Geometry: final body of the model. Coordinates: model frame, mm. A direction names the side the tool comes from. Round coordinates to 2 decimals unless told otherwise and drop trailing zeros. Loops run counter-clockwise (first coordinate to the right, second up) from the corner with the lowest first, then second, coordinate; pieces in that order, holes last. Notation, with made-up numbers: M 68,41 L 95,41 A17 cw 95,60 Z; hole C 66.5,63.25 d6. An arc over 180 degrees is marked long. Answer as a JSON object with one key per item and string values.
from build123d import *

# Parameters (mm, degrees)
F0_R     = 3.175
F0_R_2   = 3.96875
F1_DEPTH = 3.175
F2_R     = 7.9375


with BuildPart() as f1:
    # F0 (on Top) → F1 (new body)
    with BuildSketch(Plane.XY):
        with BuildLine():
            ThreePointArc((-7.9324362036, 44.7334821429), (-0.1417636831, 36.5137660501), (7.9375, 44.45))
            ThreePointArc((7.9375, 44.45), (7.9362339499, 44.5917636831), (7.9324362036, 44.7334821429))
            ThreePointArc((7.9324362036, 44.7334821429), (0, 52.3875), (-7.9324362036, 44.7334821429))
        make_face()
        with Locations((0, 44.45)):
            Circle(F0_R, mode=Mode.SUBTRACT)
        with BuildLine():
            ThreePointArc((7.9324362036, 44.7334821429), (7.9362339499, 44.5917636831), (7.9375, 44.45))
            ThreePointArc((7.9375, 44.45), (-0.1417636831, 36.5137660501), (-7.9324362036, 44.7334821429))
            Line((-7.9324362036, 44.7334821429), (-9.5189234444, 0.3401785714))
            ThreePointArc((-9.5189234444, 0.3401785714), (-6.9355783144, 6.5286582423), (-0.9144, 9.481007206))
            Line((-0.9144, 9.481007206), (9.157542126, 10.4524001899))
            Line((9.157542126, 10.4524001899), (7.9324362036, 44.7334821429))
        make_face()
        with BuildLine():
            Line((9.51892344, 0.3401786947), (9.157542126, 10.4524001899))
            Line((9.157542126, 10.4524001899), (-0.9144, 9.481007206))
            ThreePointArc((-0.9144, 9.481007206), (6.2767939568, 7.164320109), (9.51892344, 0.3401786947))
        make_face()
        with BuildLine():
            Line((62.000384, 15.5488518178), (9.157542126, 10.4524001899))
            Line((9.157542126, 10.4524001899), (9.51892344, 0.3401786947))
            ThreePointArc((9.51892344, 0.3401786947), (9.5234807388, 0.1701164813), (9.525, 0))
            ThreePointArc((9.525, 0), (6.4037475356, -7.0510738544), (-0.9144, -9.481007206))
            Line((-0.9144, -9.481007206), (62.000384, -15.5488518178))
            ThreePointArc((62.000384, -15.5488518178), (47.879, 0), (62.000384, 15.5488518178))
        make_face()
        with Locations((16.1159988493, 0)):
            Circle(F0_R, mode=Mode.SUBTRACT)
        with BuildLine():
            ThreePointArc((-0.9144, 9.481007206), (-6.9355783144, 6.5286582423), (-9.5189234444, 0.3401785714))
            ThreePointArc((-9.5189234444, 0.3401785714), (-7.1643200684, -6.2767940031), (-0.9144, -9.481007206))
            ThreePointArc((-0.9144, -9.481007206), (6.4037475356, -7.0510738544), (9.525, 0))
            ThreePointArc((9.525, 0), (9.5234807388, 0.1701164813), (9.51892344, 0.3401786947))
            ThreePointArc((9.51892344, 0.3401786947), (6.2767939568, 7.164320109), (-0.9144, 9.481007206))
        make_face()
        Circle(F0_R, mode=Mode.SUBTRACT)
        with BuildLine():
            ThreePointArc((79.121, 0), (74.0021459584, 11.5637611212), (62.000384, 15.5488518178))
            ThreePointArc((62.000384, 15.5488518178), (47.879, 0), (62.000384, -15.5488518178))
            ThreePointArc((62.000384, -15.5488518178), (74.0021459584, -11.5637611212), (79.121, 0))
        make_face()
        with Locations((63.5, 0)):
            Circle(F0_R_2, mode=Mode.SUBTRACT)
    extrude(amount=F1_DEPTH)

    # F2
    f2_edges = [f1.edges().sort_by_distance(p)[0] for p in [
        (9.157542, 10.4524, 1.5875),
    ]]
    fillet(f2_edges, radius=F2_R)


solid = f1.part
1) Ray query, line 1 (Y direction, x = 63.5, z = 1.5); line 2 (X direction, y = 1.5, z = 0.8); line 3 (X direction, y = -2.5, z = 0.65). Return the intervals inside material, ascending.
Results:
{"line 1": "-15.62 to -3.97, 3.97 to 15.62", "line 2": "-9.48 to -2.8, 2.8 to 13.32, 18.91 to 59.83, 67.17 to 79.05", "line 3": "-9.19 to -1.96, 1.96 to 14.16, 18.07 to 60.42, 66.58 to 78.92"}
2) Pull-direction query (Y, two-part tool) for faces 3 (the cylindrical face through (12.944, 0.14, 1.565)), 4 (the cylindrical face through (79.117, -0.365, 1.565)), 5 (the flat face through (24, 11, 3.175)), 6 (the cylindrical face through (0.171, 52.386, 1.565)); classes: +Y half, -Y half, draft (parallel to the pull), parting line (faces both ways), or undercut.
Results:
{"face 3": "undercut", "face 4": "parting line", "face 5": "draft", "face 6": "+Y half"}
3) Pin query (flat end, axial travel): P1, Ø4, axis at x = 10.5, y = 8, coming from the -Z side; P2, Ø5, axis at x = 0, y = 0, coming from the -Z side; P3, Ø1.5, axis at x = 15, z = 2.5, coming from the -Y side. Return the tip coordinate at first contact, or that it passes through.
Results:
{"P1": "z = 0", "P2": "through", "P3": "y = -11.09"}
4) Section query B-B (y = 46). Return the cut outline in (x, z) (3 decimals).
Results:
{"outline": "M -7.785,0 L -2.771,0 L -2.771,3.175 L -7.785,3.175 Z; M 2.771,0 L 7.785,0 L 7.785,3.175 L 2.771,3.175 Z"}
5) Reachability of faces 1 (the flat face through (40.087, 13.435, 1.565)), 2 (the cylindrical face through (1.707, 47.127, 1.565)) from +Z, -Z, +X, -X, +Y, -Y: full face, straight path, thin tool, end or side. Return the list, or none.
Results:
{"face 1": "+Z, -Z, +Y", "face 2": "+Z, -Z"}
6) Section query C-C (x = 63.5). Return the cut outline in (y, z) (3 decimals).
Results:
{"outline": "M -15.621,0 L -3.969,0 L -3.969,3.175 L -15.621,3.175 Z; M 3.969,0 L 15.621,0 L 15.621,3.175 L 3.969,3.175 Z"}
7) Section query A-A (z = 1.8). Count the separate pieces of the cut face and the enclosed holes in it, and give its area (3 significant figures).
Results:
{"separate pieces": "1", "enclosed holes": "4", "area": "2,710 mm2"}
8) Section query D-D (y = 24). Return the cut outline in (x, z) (3 decimals).
Results:
{"outline": "M -8.673,0 L 8.673,0 L 8.673,3.175 L -8.673,3.175 Z"}
